```python
from build123d import *

# Parameters (mm, degrees)
SKETCH1_W           = 120
SKETCH1_H           = 204
BOSS_EXTRUDE1_DEPTH = 30
SHELL1_T            = 8
SKETCH2_W           = 104
SKETCH2_H           = 188
CUT_EXTRUDE1_DEPTH  = 18


with BuildPart() as part:
    # Sketch1 → Boss-Extrude1 (new body)
    with BuildSketch(Plane(origin=(0, 0, 0), x_dir=(1, 0, 0), z_dir=(0, 1, 0))):
        Rectangle(SKETCH1_W, SKETCH1_H)
    extrude(amount=BOSS_EXTRUDE1_DEPTH)

    # Shell1 (no face opened: a closed hollow body)
    add(offset(amount=-SHELL1_T, mode=Mode.PRIVATE), mode=Mode.SUBTRACT)

    # Sketch2 → Cut-Extrude1 (cut)
    with BuildSketch(Plane.XZ):
        Rectangle(SKETCH2_W, SKETCH2_H)
    extrude(amount=-CUT_EXTRUDE1_DEPTH, mode=Mode.SUBTRACT)


solid = part.part
```
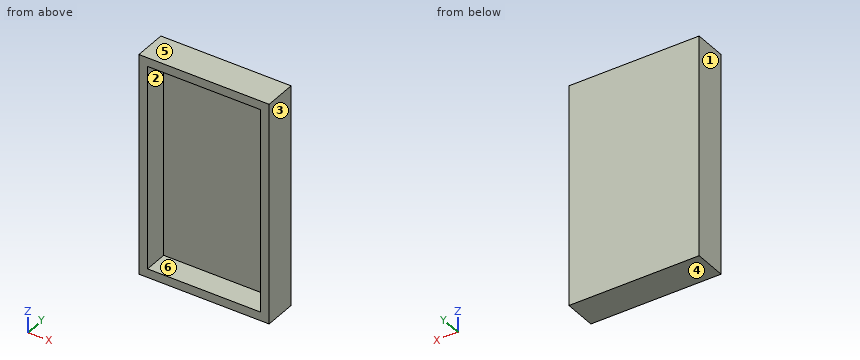
CAD build for the part. Positions are in the model's coordinates, mm. Face numbers are marked on the shaded views. A direction names the side the tool comes from. Round coordinates to 2 decimals unless told otherwise and drop trailing zeros. Order: outer loops, then holes, each group sorted by start corner. A loop starts at its lowest first (then second) coordinate and runs counter-clockwise, first axis right, second up.
Item 1: Tool access for the marked faces 1 and 2: list every direction of +Z, -Z, +X, -X, +Y, -Y with a clear straight run to the whole face (end or side of a thin tool).
Item 2: Saw through at A-A on y = 10.25. Write the cut outline in (x, z).
Item 3: Saw through at B-B on z = 52. Write the cut outline in (x, y).
Item 4: Pin check, flat tip, straight feed: pin 1 (3 mm diameter, centred on x = 29.5, z = 29, fed in from -Y). Stop position of the tip, or through.
Item 5: Saw through at C-C on x = 1. Write the cut outline in (y, z), then the cut area to 3 significant figures.
Item 6: Mould opens along Z. For the marked faces 3, 4, 5 and 6 say: pulls with the +Z half, pulls with the -Z half, needs draft (parallel to the pull), parting line crosses it, or undercut.
Item 7: Probe line 1 along X through (y, z) = (4, -63); line 2 along Z through (x, y) = (-35, 1.5); line 3 along Y through (x, z) = (-49.5, -33). List the from-to ranges inside material, lowest first.
Reported:
1. face 1: +Z, -Z, -X, +Y, -Y
1. face 2: -Y
2. outline: (-60, -102) - (60, -102) - (60, 102) - (-60, 102) - close; hole (-52, -94) - (52, -94) - (52, 94) - (-52, 94) - close
3. outline: (-60, 0) - (-52, 0) - (-52, 22) - (52, 22) - (52, 0) - (60, 0) - (60, 30) - (-60, 30) - close
4. pin 1: stops at y = 22
5. outline: (0, -102) - (30, -102) - (30, 102) - (0, 102) - (0, 94) - (22, 94) - (22, -94) - (0, -94) - close
5. area: 1,980 mm2
6. face 3: needs draft
6. face 4: pulls with the -Z half
6. face 5: pulls with the +Z half
6. face 6: undercut
7. line 1: x = -60 to -52, 52 to 60
7. line 2: z = -102 to -94, 94 to 102
7. line 3: y = 22 to 30
